from build123d import *

# Parameters (mm, degrees)
F0_R        = 2.75
F0_R_2      = 13
F0_R_3      = 10.75
F1_DEPTH    = 30
F2_START    = 30
F2_DEPTH    = 14
F3_S5_R     = 13
F3_T6_DEPTH = 23
F4_SIZE     = 5
F5_T1_DEPTH = 117.8673195186
F5_T3_DEPTH = 120.3673195186


# Not quite as in the source:
# - a fillet or chamfer that OpenCascade refuses, or shapes differently, is made with other operations: its cross-section is extruded or revolved along the edge and cut away or added


with BuildPart() as f1:
    # F0 (on Top) → F1 (new body)
    with BuildSketch(Plane.XY):
        Polygon((0, 28.3), (0, 15), (-15, 15), (-15, -14), (-7.5, -14), (-7.5, -28.3), (0, -28.3), (15, -28.3), (15, 15), (15, 28.3), align=None)
        with Locations((0, -20.5)):
            Circle(F0_R, mode=Mode.SUBTRACT)
        Circle(F0_R_2, mode=Mode.SUBTRACT)
        Circle(F0_R_2)
        Circle(F0_R_3, mode=Mode.SUBTRACT)
    extrude(amount=F1_DEPTH)

    # F0 (on Top) → F2 (join)
    with BuildSketch(Plane.XY.offset(F2_START)):
        Polygon((0, 28.3), (0, 15), (-15, 15), (-15, -14), (-7.5, -14), (-7.5, -28.3), (0, -28.3), (15, -28.3), (15, 15), (15, 28.3), align=None)
        with Locations((0, -20.5)):
            Circle(F0_R, mode=Mode.SUBTRACT)
        Circle(F0_R_2, mode=Mode.SUBTRACT)
    extrude(amount=F2_DEPTH)

    # F3: chamfer of 4.5 on 1 edges, made by hand


with BuildPart() as f3_tool2:
    # F3_s3 → F3_t4 (revolve)
    with BuildSketch(Plane.XZ):
        Polygon((10.75, 25.5), (15.25, 30), (10.75, 30), align=None)
    revolve(axis=Axis((0, 0, 30), (0, 0, 1)))

    # F3_s5 → F3_t6 (intersect, symmetric)
    with BuildSketch(Plane.XY.offset(27.8)):
        Circle(F3_S5_R)
    extrude(amount=F3_T6_DEPTH, both=True, mode=Mode.INTERSECT)


with BuildPart() as f1_1:
    add(f1.part)

    # F3_t1: cut F3_tool2
    add(f3_tool2.part, mode=Mode.SUBTRACT)

    # F4
    f4_edges = [f1_1.edges().sort_by_distance(p)[0] for p in [
        (15, -28.3, 22),
    ]]
    chamfer(f4_edges, length=F4_SIZE)

    # F5: chamfer of 20 on 2 edges, made by hand

    # F5_s2 → F5_t1 (cut)
    with BuildSketch(Plane.YZ.offset(-51.4336597593)):
        Polygon((28.3, 24), (8.3, 44), (28.3, 44), align=None)
    extrude(amount=F5_T1_DEPTH, mode=Mode.SUBTRACT)

    # F5_s4 → F5_t3 (cut)
    with BuildSketch(Plane.YZ.offset(-58.9336597593)):
        Polygon((-28.3, 24), (-8.3, 44), (-28.3, 44), align=None)
    extrude(amount=F5_T3_DEPTH, mode=Mode.SUBTRACT)


solid = f1_1.part
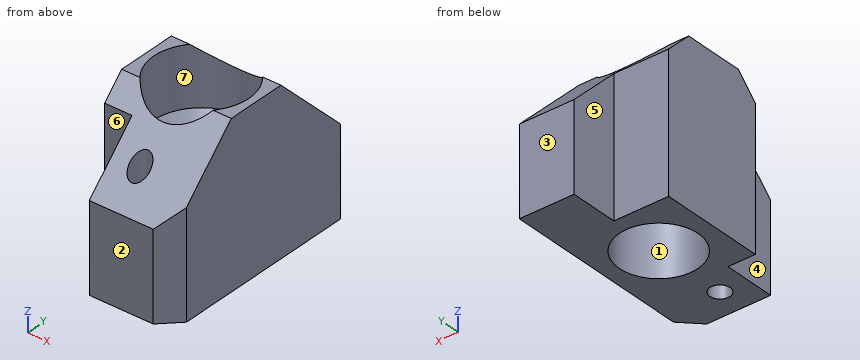
The model under review builds one solid part; all positions refer to its coordinate system, in mm. Face numbers are marked on the shaded views. A direction names the side the tool comes from. Round coordinates to 2 decimals unless told otherwise and drop trailing zeros. Loops run counter-clockwise (first coordinate to the right, second up) from the corner with the lowest first, then second, coordinate; pieces in that order, holes last. Notation, with made-up numbers: (50, 87) -> (88, 87) arc R23 ccw to (88, 113) -> close; hole circle Ø1 at (18, 7.5). An arc over 180 degrees is marked (long way). Write item = value, one per line. Start each with the question number.
Item 1: To check wall thickness, follow L1, parallel to X at y = 0, z = 34.75; L2, parallel to Y at x = -1.5, z = 16; L3, parallel to X at y = -16.5, z = 22. State the ranges of each line that lie inside material, in increasing order.
Item 2: Take a section at A-A on y = 0. Give the boundary of the cut face in (x, z), plus the area to 3 significant figures.
Item 3: Take a section at C-C on y = -20.5. Give the boundary of the cut face in (x, z).
Item 4: Mouldability with a two-part tool opening along Y and no side actions: class the marked faces 1, 2, 3 and 4 as released by +Y, released by -Y, zero draft, split by the parting line, or undercut.
Item 5: Take a section at B-B on z = 22. Give the boundary of the cut face in (x, y).
Item 6: Take a section at D-D on y = 14. Give the boundary of the cut face in (x, z), plus the area to 3 significant figures.
Item 7: For the marked faces 5, 6 and 7, list the 3-axis set-ups (+Z, -Z, +X, -X, +Y, -Y) from which the entire face can be reached by the end or side of a thin tool; tool diameter is ignored.
Item 8: Insertion check: pin 1 (12 mm diameter, centred on x = -1.5, z = 32.5, fed in from -Y); pin 2 (7.5 mm diameter, centred on x = -6, z = 15.5, fed in from +Y); pin 3 (10 mm diameter, centred on y = 22.5, z = 25.5, fed in from -X). Each pin has a flat end and moves straight along its axis. Give the tip position at first contact, or say it passes through.
Result:
q1.L1 = -15 to -13, 13 to 15
q1.L2 = -28.3 to -22.8, -18.2 to -10.64, 10.64 to 15
q1.L3 = -7.5 to 15
q2.outline = (-15, 0) -> (-10.75, 0) -> (-10.75, 25.5) -> (-13, 27.75) -> (-13, 44) -> (-15, 44) -> close; (10.75, 0) -> (15, 0) -> (15, 44) -> (13, 44) -> (13, 27.75) -> (10.75, 25.5) -> close
q2.area = 296 mm²
q3.outline = (-7.5, 0) -> (-2.75, 0) -> (-2.75, 31.8) -> (-7.5, 31.8) -> close; (2.75, 0) -> (15, 0) -> (15, 31.8) -> (2.75, 31.8) -> close
q4.face_1 = undercut
q4.face_2 = released by -Y
q4.face_3 = released by +Y
q4.face_4 = zero draft
q5.outline = (-15, -14) -> (-7.5, -14) -> (-7.5, -28.3) -> (10, -28.3) -> (15, -23.3) -> (15, 28.3) -> (0, 28.3) -> (0, 15) -> (-15, 15) -> close; hole circle Ø21.5 at (0, 0); hole circle Ø5.5 at (0, -20.5)
q6.outline = (-15, 0) -> (15, 0) -> (15, 38.3) -> (-15, 38.3) -> close
q6.area = 1,150 mm²
q7.face_5 = +Z, -Z, -X, +Y
q7.face_6 = +Z, -Z, -X, -Y
q7.face_7 = +Z
q8.pin_1 = -25.8
q8.pin_2 = 15
q8.pin_3 = 0
